Autodesk Inventor part; units mm, degrees
ref_plane "YZ Plane" through (0, 0, 0) normal (1, 0, 0) x (0, 1, 0)
ref_plane "XZ Plane" through (0, 0, 0) normal (0, 1, 0) x (-1, 0, 0)
ref_plane "XY Plane" through (0, 0, 0) normal (0, 0, 1) x (1, 0, 0)
sketch "Sketch1" plane through (0, 0, 0) normal (0, 1, 0) x (-1, 0, 0)
  line L0 (10, -45) -> (-10, -45)
  line L1 (-10, -45) -> (-10, 45)
  line L2 (-10, 45) -> (10, 45)
  line L3 (10, 45) -> (10, -45)
  point P0 (0, 0)
  dimension "d0" = 20
  dimension "d1" = 90
  dimension "d2" = 45
  dimension "d3" = 10
extrude "Plate1" add sketch "Sketch1" along normal blind 1.5
sketch "Sketch2" plane through (0, 0, 0) normal (0, -1, 0) x (1, 0, 0)
  circle A0 centre (0, 42) radius 0.7835
  circle A1 centre (-7, 35) radius 0.7835
  circle A2 centre (0, 28) radius 0.7835
  circle A3 centre (7, 35) radius 0.7835
  circle A4 centre (0, -28) radius 0.7835
  circle A5 centre (-7, -35) radius 0.7835
  circle A6 centre (0, -42) radius 0.7835
  circle A7 centre (7, -35) radius 0.7835
  point P0 (0, 0)
hole "Hole1" at (0, 0, 42) at (-7, 0, 35) at (0, 0, 28) at (7, 0, 35) at (0, 0, -28) at (-7, 0, -35) at (0, 0, -42) at (7, 0, -35) direction (0, 1, 0) diameter 2.1 depth 1.5
sketch "Sketch3" plane through (0, 1.5, 0) normal (0, 1, 0) x (1, 0, 0)
  arc A0 (10, 35) -> (-10, 35) centre (0, 35) ccw
  arc A1 (-10, -35) -> (10, -35) centre (0, -35) ccw
  line L0 (-10, 35) -> (-10, -35)
  line L1 (10, 35) -> (10, -35)
  line L2 (10, 45) -> (10, -45)
  line L3 (-10, 45) -> (10, 45)
  line L4 (10, 45) -> (10, -45)
  line L5 (10, -45) -> (-10, -45)
  line L6 (-10, -45) -> (-10, 45)
  point P0 (0, 0)
  point P1 (0, 45)
  point P2 (10, 35)
  point P3 (-10, -35)
  point P4 (0, -45)
  point P5 (10, -35)
  dimension "d12" = 35
  dimension "d13" = 35
  dimension "d14" = 10
  dimension "d15" = 10
  dimension "d16" = 10
  dimension "d17" = 20
  dimension "d18" = 90
extrude "Extrusion1" cut sketch "Sketch3" against normal blind 10 contours A0 L3 L2 | A0 L6 L3 | L2 L5 A1 | L5 L6 A1
equation "\"d10\" = Thickness"
equation "\"d4\" = Thickness"
equation "\"BendReliefWidth\" = Thickness"
equation "\"BendReliefDepth\" = 0.5 * Thickness"
equation "\"CornerReliefSize\" = 4 * Thickness"
equation "\"MinimumRemnant\" = 2 * Thickness"
equation "\"TransitionRadius\" = BendRadius"
equation "\"JacobiRadiusSize\" = BendRadius"
equation "\"GapSize\" = Thickness"
properties part number "axis_10_11-connector_frame" material "Aluminum 6061-AHC"
Source: CAD feature listing. Evaluate the final solid. Frame: model axes, mm. Round coordinates to 2 decimals unless told otherwise and drop trailing zeros. Write each loop counter-clockwise with the first axis right and the second up, starting at its lowest first coordinate (ties: lowest second). Pieces come first, ordered by that corner, then holes. Notation, with made-up numbers: (26.25, 43) - (44.25, 43) arc R25 ccw to (44.25, 77) - close; hole circle Ø5 at (-8, -36.75). An arc over 180 degrees is marked (long way). Use CSV: the item, a comma, the result in double quotes. Start each with the question number.
(1) Cut plane D-D, the plane z = -42. Return loops of the section in (x, y).
(2) Material intervals for probe 1 along Z at (x, y) = (0, 0.3); probe 2 along X at (y, z) = (1.2, -35); probe 3 along Z at (x, y) = (-7, 0.6), sorted ascending. Write a range as [from, to].
(3) Cut plane B-B, the plane y = 1. Give the number of separate pieces and of enclosed holes in the cut face, and give its area (3 significant figures).
(4) Mould query, pull axis X, two halves, no side actions, for faces 1 (the face through (0, 1, 45)), 2 (the face through (-0.05, 0.76, 43.05)), 3 (the face through (-10, 1, 0)). Classes: pulls with the +X half, pulls with the -X half, needs draft (parallel to the pull), parting line crosses it, or undercut.
(5) Cut plane A-A, the plane z = -28. Return loops of the section in (x, y).
(6) First-contact query: pin 1 Ø1.3 at (x, z) = (7, 35) entering from -Y. Flat tip, straight axial feed; report the tip coordinate or a pass-through.
(7) Cut plane C-C, the plane x = 7. Return loops of the section in (y, z).
Geometry says:
1,outline,"(-7.14, 0) - (-1.05, 0) - (-1.05, 1.5) - (-7.14, 1.5) - close; (1.05, 0) - (7.14, 0) - (7.14, 1.5) - (1.05, 1.5) - close"
2,probe 1,"[-45, -43.05], [-40.95, -29.05], [-26.95, 26.95], [29.05, 40.95], [43.05, 45]"
2,probe 2,"[-10, -8.05], [-5.95, 5.95], [8.05, 10]"
2,probe 3,"[-42.14, -36.05], [-33.95, 33.95], [36.05, 42.14]"
3,separate pieces,"1"
3,enclosed holes,"8"
3,area,"1,690 mm²"
4,face 1,"parting line crosses it"
4,face 2,"undercut"
4,face 3,"pulls with the -X half"
5,outline,"(-10, 0) - (-1.05, 0) - (-1.05, 1.5) - (-10, 1.5) - close; (1.05, 0) - (10, 0) - (10, 1.5) - (1.05, 1.5) - close"
6,pin 1,"through"
7,outline,"(0, -42.14) - (1.5, -42.14) - (1.5, -36.05) - (0, -36.05) - close; (0, -33.95) - (1.5, -33.95) - (1.5, 33.95) - (0, 33.95) - close; (0, 36.05) - (1.5, 36.05) - (1.5, 42.14) - (0, 42.14) - close"
